Autodesk Inventor part; units mm, degrees
ref_plane "MSC_PF1" through (0, 0, 0) normal (0, 1, 0) x (-1, 0, 0)
ref_plane "MSC_PT1" through (0, 0, 63.7798) normal (0, 0, -1) x (-1, 0, 0)
ref_plane "YZ Plane" through (0, 0, 0) normal (1, 0, 0) x (0, 1, 0)
sketch "Sketch2" plane through (0, 0, 0) normal (0, 1, 0) x (-1, 0, 0)
  line L0 (0, 63.7798) -> (0, -36.2202)
  line L1 (0, -36.2202) -> (7, -36.2202)
  line L2 (8, -35.2202) -> (8, 1.7798)
  line L3 (8, 1.7798) -> (7.25, 3.0788)
  line L4 (7.25, 3.0788) -> (7.25, 63.7798)
  line L5 (7.25, 63.7798) -> (0, 63.7798)
  line L6 (7, -36.2202) -> (8, -35.2202)
  line L7 (8, -36.2202) -> (8, -37.6344)
  line L8 (0, -57.9172) -> (0, 84.0627)
  dimension "Ds" = 14.5
  dimension "NND" = 16
  dimension "b" = 38
  dimension "d3" = 30
  dimension "d5" = 45
  dimension "PTC" = 2
  dimension "NLG" = 100
revolve "Revolution1" add sketch "Sketch2" angle 360 about axis through (0, 0, 63.7798) along (0, 0, -1)
sketch "Sketch3" plane through (0, 0, 63.7798) normal (0, 0, 1) x (1, 0, 0)
  circle A0 centre (0, 0) radius 7.25
  line L0 (0, 12) -> (6.9282, 12)
  line L1 (6.9282, 12) -> (13.8564, 0)
  line L2 (13.8564, 0) -> (0, 0)
  line L3 (0, 0) -> (0, 12)
  line L4 (0, 12) -> (-6.9282, 12)
  line L5 (-6.9282, 12) -> (-13.8564, 0)
  line L6 (0, -12) -> (6.9282, -12)
  line L7 (6.9282, -12) -> (13.8564, 0)
  line L8 (-6.9282, -12) -> (-13.8564, 0)
  line L9 (0, -12) -> (-6.9282, -12)
  dimension "d9" = 60
  dimension "ParS" = 24
  dimension "msp_d11" = 24
extrude "Extrusion1" add sketch "Sketch3" along normal blind 10
sketch "Sketch4" plane through (0, 0, 0) normal (0, 1, 0) x (-1, 0, 0)
  line L0 (-12, 73.7798) -> (-13.8564, 73.7798)
  line L1 (-13.8564, 73.7798) -> (-13.8564, 72.708)
  line L2 (-13.8564, 72.708) -> (-12, 73.7798)
  line L3 (0, 17.8585) -> (0, 83.1)
  line L4 (0, 28.2505) -> (0, 27.1787)
  line L5 (-13.8564, 63.7798) -> (-13.8564, 73.7798)
  line L6 (-6.9282, 73.7798) -> (-13.8564, 73.7798)
  dimension "d14" = 30
  dimension "msp_d15" = 24
revolve "Revolution2" cut sketch "Sketch4" angle 360 about axis through (0, 0, 28.2505) along (0, 0, -1)
sketch "Sketch5" plane through (0, 0, 73.7798) normal (0, 0, 1) x (1, 0, 0)
  arc A0 (10.3923, 6) -> (0, 12) centre (0, 0) ccw
  circle A1 centre (0, 0) radius 9
  dimension "d27" = 18
extrude "Extrusion2" cut sketch "Sketch5" against normal blind 2
thread "Thread1"
ref_plane "MSC_PF1" through (0, 0, 0) normal (0, 1, 0) x (-1, 0, 0)
ref_plane "MSC_PT1" through (0, 0, 63.7798) normal (0, 0, -1) x (-1, 0, 0)
fillet "Fillet1" radius 0.6 1 edges at (7.25, 0, 63.7798)
equation "\"msp_d11\" = ParS"
equation "\"msp_d15\" = ParS"
equation "\"d27\" = 0.75 * ParS"
equation "\"d28\" = 0.2 * ParK"
equation "\"d30\" = r"
equation "\"msp_d17\" = b"
equation "\"r\" = 0.6"
equation "\"THREADDIA\" = NND"
properties part number "NF EN ISO 4015 - M16x100" material "Stainless Steel, 440C"
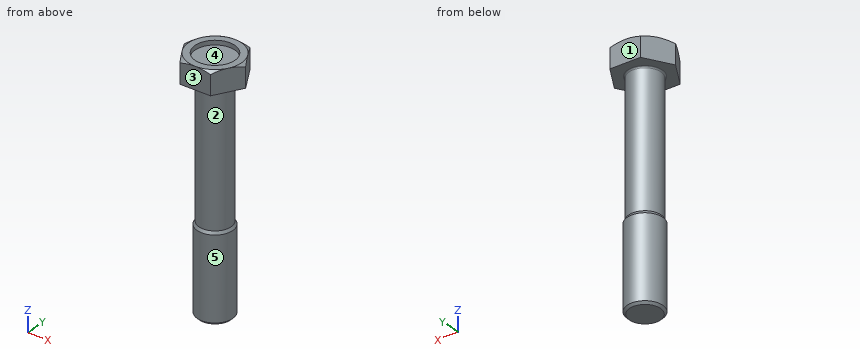
Work out the finished part from the listing and answer in its coordinate system (mm). Face numbers are marked on the shaded views. A direction names the side the tool comes from. Round coordinates to 2 decimals unless told otherwise and drop trailing zeros. Write each loop counter-clockwise with the first axis right and the second up, starting at its lowest first coordinate (ties: lowest second). Pieces come first, ordered by that corner, then holes.
1) Straight lines are drawn through the part: line 1 (Y direction, x = 0, z = 72.9); line 2 (X direction, y = 0.5, z = -7.5); line 3 (Z direction, x = 3.5, y = -2). For each, find the intervals that lie inside material, in ascending order.
2) A cutting plane is placed at B-B (z = 17.5). Give the vertices of the cut face in (x, y).
3) A cutting plane is placed at A-A (z = 66). Give the vertices of the cut face in (x, y), plus the area to 3 significant figures.
4) The mould has two halves that part along Y. Classify the marked faces 3, 4 and 5: pulls with the +Y half, pulls with the -Y half, needs draft (parallel to the pull), parting line crosses it, or undercut.
5) A cutting plane is placed at C-C (z = -23.5). Give the vertices of the cut face in (x, y), plus the area to 3 significant figures.
6) A tool of negligible diameter and unlimited length cuts with its end or side. For the marked faces 1 and 2, from which of +Z, -Z, +X, -X, +Y, -Y can it reach the whole face along a straight path? Write none if from no direction.
7) Given pin 1 Ø10 at (x, z) = (0, -11.5) entering from -Y; pin 2 Ø5.5 at (x, y) = (-3, 4) entering from +Z; pin 3 Ø10 at (y, z) = (2.5, 29.5) entering from +X, each flat-ended and moving along its own axis, determine where each tip first touches the part or whether it passes through.
Completed:
1. line 1: y = -12 to -9, 9 to 12
1. line 2: x = -7.98 to 7.98
1. line 3: z = -36.22 to 71.78
2. outline: circle Ø14.5 at (0, 0)
3. outline: (-13.86, 0) - (-6.93, -12) - (6.93, -12) - (13.86, 0) - (6.93, 12) - (-6.93, 12) - close
3. area: 499 mm2
4. face 3: pulls with the -Y half
4. face 4: undercut
4. face 5: parting line crosses it
5. outline: circle Ø16 at (0, 0)
5. area: 201 mm2
6. face 1: +Z, -Z, +X, -X, +Y
6. face 2: none
7. pin 1: stops at y = -8
7. pin 2: stops at z = 71.78
7. pin 3: stops at x = 7.25
